Geometry: final body of the model. Coordinates: model frame, mm. Coordinates: 2 decimals unless noted, no trailing zeros. Write each loop counter-clockwise with the first axis right and the second up, starting at its lowest first coordinate (ties: lowest second). Pieces come first, ordered by that corner, then holes. Notation, with made-up numbers: (-34, -33) - (0, -33) arc R15 ccw to (0, -13) - close; hole circle Ø9 at (-7, -38). An arc over 180 degrees is marked (long way). Answer as a JSON object with one key per item and string values. Group by question number.
Item 1: Section B-B on y = 0.45. Return loops of the section in (x, z).
Item 2: Section C-C on z = 7. Return loops of the section in (x, y).
Item 3: Line query: line 1 along X through (y, z) = (0.35, -7); line 2 along Y through (x, z) = (-3.25, -7.75); line 3 along X through (y, z) = (-0.45, -2.25). Output: solid intervals per line, ascending. Write a range as from..to.
Item 4: First-contact query: pin 1 Ø5 at (x, z) = (-7, 7) entering from -Y; pin 2 Ø0.5 at (y, z) = (-0.5, 0.5) entering from +X; pin 3 Ø0.5 at (x, y) = (-0.5, -0.5) entering from -Z. Flat tips, straight axial feed; report the tip coordinate or a pass-through.
Item 5: Section A-A on z = -7. Return loops of the section in (x, y).
Item 6: Section D-D on x = 7. Return loops of the section in (y, z), and give its area (3 significant figures).
```python
from build123d import *

# Parameters (mm, degrees)
SKETCH1_R           = 1.5
BOSS_EXTRUDE1_DEPTH = 1.6
SKETCH2_W           = 4.3
SKETCH2_H           = 5.2
BOSS_EXTRUDE2_DEPTH = 1


with BuildPart() as part:
    # Sketch1 → Boss-Extrude1 (new body)
    with BuildSketch(Plane(origin=(0, 0, 0), x_dir=(1, 0, 0), z_dir=(0, 1, 0))):
        with BuildLine():
            Line((8.25, 11.25), (-8.25, 11.25))
            ThreePointArc((-8.25, 11.25), (-10.371320344, 10.371320344), (-11.25, 8.25))
            Line((-11.25, 8.25), (-11.25, -8.25))
            ThreePointArc((-11.25, -8.25), (-10.371320344, -10.371320344), (-8.25, -11.25))
            Line((-8.25, -11.25), (8.25, -11.25))
            ThreePointArc((8.25, -11.25), (10.371320344, -10.371320344), (11.25, -8.25))
            Line((11.25, -8.25), (11.25, 8.25))
            ThreePointArc((11.25, 8.25), (10.371320344, 10.371320344), (8.25, 11.25))
        make_face()
        with Locations(Location((7, 7, 0), (0, 0, 270))):
            Circle(SKETCH1_R, mode=Mode.SUBTRACT)
        with Locations(Location((-7, 7, 0), (0, 0, 90))):
            Circle(SKETCH1_R, mode=Mode.SUBTRACT)
        with Locations(Location((-7, -7, 0), (0, 0, 270))):
            Circle(SKETCH1_R, mode=Mode.SUBTRACT)
    extrude(amount=BOSS_EXTRUDE1_DEPTH)

    # Sketch2 → Boss-Extrude2 (add)
    with BuildSketch(Plane.XZ):
        Rectangle(SKETCH2_W, SKETCH2_H)
    extrude(amount=BOSS_EXTRUDE2_DEPTH)


solid = part.part
```
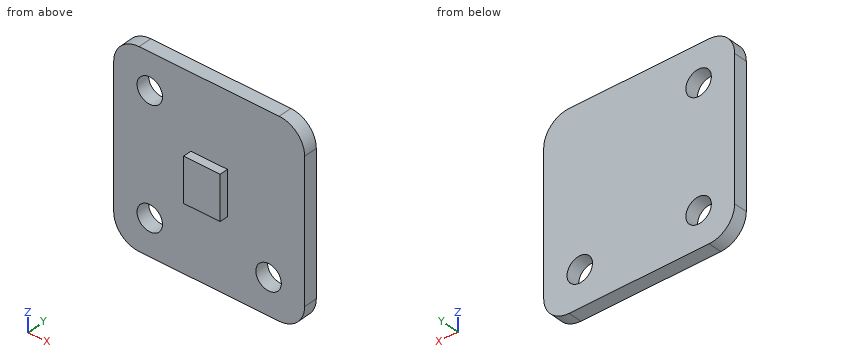
Checks:
{
 "1": {"outline": "(-11.25, -8.25) arc R3 ccw to (-8.25, -11.25) - (8.25, -11.25) arc R3 ccw to (11.25, -8.25) - (11.25, 8.25) arc R3 ccw to (8.25, 11.25) - (-8.25, 11.25) arc R3 ccw to (-11.25, 8.25) - close; hole circle Ø3 at (-7, -7); hole circle Ø3 at (-7, 7); hole circle Ø3 at (7, -7)"},
 "2": {"outline": "(-11.25, 0) - (-8.5, 0) - (-8.5, 1.6) - (-11.25, 1.6) - close; (-5.5, 0) - (11.25, 0) - (11.25, 1.6) - (-5.5, 1.6) - close"},
 "3": {"line 1": "-11.25..-8.5, -5.5..5.5, 8.5..11.25", "line 2": "0..1.6", "line 3": "-2.15..2.15"},
 "4": {"pin 1": "y = 0", "pin 2": "x = 2.15", "pin 3": "z = -2.6"},
 "5": {"outline": "(-11.25, 0) - (-8.5, 0) - (-8.5, 1.6) - (-11.25, 1.6) - close; (-5.5, 0) - (5.5, 0) - (5.5, 1.6) - (-5.5, 1.6) - close; (8.5, 0) - (11.25, 0) - (11.25, 1.6) - (8.5, 1.6) - close"},
 "6": {"outline": "(0, -11.25) - (1.6, -11.25) - (1.6, -8.5) - (0, -8.5) - close; (0, -5.5) - (1.6, -5.5) - (1.6, 11.25) - (0, 11.25) - close", "area": "31.2 mm^2"}
}
